```python
from build123d import *

# Parameters (mm, degrees)
BOSS_EXTRUDE1_DEPTH = 36.5
BOSS_EXTRUDE2_DEPTH = 40.35
SKETCH1_4_W         = 22.175
SKETCH1_4_H         = 49.125448028
SKETCH1_4_W_2       = 8.7
SKETCH1_4_H_2       = 18.8
BOSS_EXTRUDE3_DEPTH = 25.8
SKETCH1_5_W         = 8.7
SKETCH1_5_H         = 18.8
BOSS_EXTRUDE4_DEPTH = 20.8
SKETCH1_6_W         = 26.5
SKETCH1_6_H         = 17
BOSS_EXTRUDE5_DEPTH = 7.2
SKETCH1_7_W         = 26.5
SKETCH1_7_H         = 16.1
BOSS_EXTRUDE6_DEPTH = 10
SKETCH1_8_W         = 26.5
SKETCH1_8_H         = 16.1
SKETCH1_8_H_2       = 17
SKETCH1_8_W_2       = 18
SKETCH1_8_H_3       = 43.5
SKETCH1_8_W_3       = 79.7
SKETCH1_8_H_4       = 2.437275986
BOSS_EXTRUDE7_DEPTH = 18.5
SKETCH1_9_W         = 79.7
SKETCH1_9_H         = 2.437275986
SKETCH1_9_W_2       = 26.5
SKETCH1_9_H_2       = 16.1
SKETCH1_9_H_3       = 17
SKETCH1_9_W_3       = 18
SKETCH1_9_H_4       = 43.5
SKETCH1_9_W_4       = 22.175
SKETCH1_9_H_5       = 49.125448028
SKETCH1_9_W_5       = 8.7
SKETCH1_9_H_6       = 18.8
BOSS_EXTRUDE8_DEPTH = 2
BOSS_EXTRUDE9_DEPTH = 2


with BuildPart() as part:
    # Sketch1 → Boss-Extrude1 (new body)
    with BuildSketch(Plane(origin=(0, 0, 0), x_dir=(1, 0, 0), z_dir=(0, 1, 0))):
        Polygon((-41.85, -51), (-39.85, -51), (-39.85, -48.562724014), (-39.85, -28.312724014), (-39.85, 48.562724014), (17.675, 48.562724014), (39.85, 48.562724014), (39.85, -0.562724014), (39.85, -48.562724014), (39.85, -51), (41.85, -51), (41.85, 51), (-41.85, 51), align=None)
    extrude(amount=BOSS_EXTRUDE1_DEPTH)

    # Sketch1_3 → Boss-Extrude2 (add)
    with BuildSketch(Plane(origin=(0, 0, 0), x_dir=(1, 0, 0), z_dir=(0, 1, 0))):
        Polygon((43.85, -51), (41.85, -51), (41.85, 51), (-41.85, 51), (-41.85, -51), (-43.85, -51), (-43.85, 53), (43.85, 53), align=None)
    extrude(amount=BOSS_EXTRUDE2_DEPTH)

    # Sketch1_4 → Boss-Extrude3 (add)
    with BuildSketch(Plane(origin=(0, 0, 0), x_dir=(1, 0, 0), z_dir=(0, 1, 0))):
        with Locations((28.7625, 24)):
            Rectangle(SKETCH1_4_W, SKETCH1_4_H)
        with Locations((28.7625, 24)):
            Rectangle(SKETCH1_4_W_2, SKETCH1_4_H_2, mode=Mode.SUBTRACT)
    extrude(amount=BOSS_EXTRUDE3_DEPTH)

    # Sketch1_5 → Boss-Extrude4 (add)
    with BuildSketch(Plane(origin=(0, 0, 0), x_dir=(1, 0, 0), z_dir=(0, 1, 0))):
        with Locations((28.7625, 24)):
            Rectangle(SKETCH1_5_W, SKETCH1_5_H)
    extrude(amount=BOSS_EXTRUDE4_DEPTH)



with BuildPart() as body_2:
    # Sketch1_6 → Boss-Extrude5 (new body)
    with BuildSketch(Plane(origin=(0, 0, 0), x_dir=(1, 0, 0), z_dir=(0, 1, 0))):
        with Locations((4.25, -38.812724014)):
            Rectangle(SKETCH1_6_W, SKETCH1_6_H)
    extrude(amount=BOSS_EXTRUDE5_DEPTH)


with BuildPart() as body_3:
    # Sketch1_7 → Boss-Extrude6 (new body)
    with BuildSketch(Plane(origin=(0, 0, 0), x_dir=(1, 0, 0), z_dir=(0, 1, 0))):
        with Locations((-24.425, -38.812724014)):
            Rectangle(SKETCH1_7_W, SKETCH1_7_H)
    extrude(amount=BOSS_EXTRUDE6_DEPTH)


with BuildPart() as part_1:
    add(part.part)

    add(body_2.part)  # Boss-Extrude7 merges body 2

    add(body_3.part)  # Boss-Extrude7 merges body 3
    # Sketch1_8 → Boss-Extrude7 (add)
    # profile 1 of 2: a face of its own
    with BuildSketch(Plane(origin=(0, 0, 0), x_dir=(1, 0, 0), z_dir=(0, 1, 0))):
        Polygon((-39.85, -28.312724014), (-39.85, -48.562724014), (39.85, -48.562724014), (39.85, -0.562724014), (17.675, -0.562724014), (17.675, -28.312724014), align=None)
        with Locations((-24.425, -38.812724014)):
            Rectangle(SKETCH1_8_W, SKETCH1_8_H, mode=Mode.SUBTRACT)
        with Locations((4.25, -38.812724014)):
            Rectangle(SKETCH1_8_W, SKETCH1_8_H_2, mode=Mode.SUBTRACT)
        with Locations((28.675, -25.562724014)):
            Rectangle(SKETCH1_8_W_2, SKETCH1_8_H_3, mode=Mode.SUBTRACT)
    # profile 2 of 2: a face of its own
    with BuildSketch(Plane(origin=(0, 0, 0), x_dir=(1, 0, 0), z_dir=(0, 1, 0))):
        with Locations((0, -49.781362007)):
            Rectangle(SKETCH1_8_W_3, SKETCH1_8_H_4)
    extrude(amount=BOSS_EXTRUDE7_DEPTH)

    # Sketch1_9 → Boss-Extrude8 (add)
    # profile 1 of 10: a face of its own
    with BuildSketch(Plane(origin=(0, 0, 0), x_dir=(1, 0, 0), z_dir=(0, 1, 0))):
        with Locations((0, -49.781362007)):
            Rectangle(SKETCH1_9_W, SKETCH1_9_H)
    # profile 2 of 10: a face of its own
    with BuildSketch(Plane(origin=(0, 0, 0), x_dir=(1, 0, 0), z_dir=(0, 1, 0))):
        Polygon((43.85, -51), (41.85, -51), (41.85, 51), (-41.85, 51), (-41.85, -51), (-43.85, -51), (-43.85, 53), (43.85, 53), align=None)
    # profile 3 of 10: a face of its own
    with BuildSketch(Plane(origin=(0, 0, 0), x_dir=(1, 0, 0), z_dir=(0, 1, 0))):
        Polygon((-41.85, -51), (-39.85, -51), (-39.85, -48.562724014), (-39.85, -28.312724014), (-39.85, 48.562724014), (17.675, 48.562724014), (39.85, 48.562724014), (39.85, -0.562724014), (39.85, -48.562724014), (39.85, -51), (41.85, -51), (41.85, 51), (-41.85, 51), align=None)
    # profile 4 of 10: a face of its own
    with BuildSketch(Plane(origin=(0, 0, 0), x_dir=(1, 0, 0), z_dir=(0, 1, 0))):
        Polygon((-39.85, -28.312724014), (-39.85, -48.562724014), (39.85, -48.562724014), (39.85, -0.562724014), (17.675, -0.562724014), (17.675, -28.312724014), align=None)
        with Locations((-24.425, -38.812724014)):
            Rectangle(SKETCH1_9_W_2, SKETCH1_9_H_2, mode=Mode.SUBTRACT)
        with Locations((4.25, -38.812724014)):
            Rectangle(SKETCH1_9_W_2, SKETCH1_9_H_3, mode=Mode.SUBTRACT)
        with Locations((28.675, -25.562724014)):
            Rectangle(SKETCH1_9_W_3, SKETCH1_9_H_4, mode=Mode.SUBTRACT)
    # profile 5 of 10: a face of its own
    with BuildSketch(Plane(origin=(0, 0, 0), x_dir=(1, 0, 0), z_dir=(0, 1, 0))):
        with Locations((-24.425, -38.812724014)):
            Rectangle(SKETCH1_9_W_2, SKETCH1_9_H_2)
    # profile 6 of 10: a face of its own
    with BuildSketch(Plane(origin=(0, 0, 0), x_dir=(1, 0, 0), z_dir=(0, 1, 0))):
        with Locations((4.25, -38.812724014)):
            Rectangle(SKETCH1_9_W_2, SKETCH1_9_H_3)
    # profile 7 of 10: a face of its own
    with BuildSketch(Plane(origin=(0, 0, 0), x_dir=(1, 0, 0), z_dir=(0, 1, 0))):
        with Locations((28.7625, 24)):
            Rectangle(SKETCH1_9_W_4, SKETCH1_9_H_5)
        with Locations((28.7625, 24)):
            Rectangle(SKETCH1_9_W_5, SKETCH1_9_H_6, mode=Mode.SUBTRACT)
    # profile 8 of 10: a face of its own
    with BuildSketch(Plane(origin=(0, 0, 0), x_dir=(1, 0, 0), z_dir=(0, 1, 0))):
        with Locations((28.7625, 24)):
            Rectangle(SKETCH1_9_W_5, SKETCH1_9_H_6)
    # profile 9 of 10: a face of its own
    with BuildSketch(Plane(origin=(0, 0, 0), x_dir=(1, 0, 0), z_dir=(0, 1, 0))):
        Polygon((-39.85, 48.562724014), (-39.85, -28.312724014), (17.675, -28.312724014), (17.675, -0.562724014), (17.675, 48.562724014), align=None)
    # profile 10 of 10: a face of its own
    with BuildSketch(Plane(origin=(0, 0, 0), x_dir=(1, 0, 0), z_dir=(0, 1, 0))):
        with Locations((28.675, -25.562724014)):
            Rectangle(SKETCH1_9_W_3, SKETCH1_9_H_4)
    extrude(amount=-BOSS_EXTRUDE8_DEPTH)

    # Sketch2 → Boss-Extrude9 (add)
    with BuildSketch(Plane(origin=(0, 40.35, 0), x_dir=(1, 0, 0), z_dir=(0, 1, 0))):
        Polygon((-41.85, -51), (-41.85, 51), (41.85, 51), (41.85, -51), (39.85, -51), (39.85, 49), (-39.85, 49), (-39.85, -51), align=None)
    extrude(amount=-BOSS_EXTRUDE9_DEPTH)


solid = part_1.part
```
Geometry: final body of the model. Coordinates: model frame, mm. A direction names the side the tool comes from. Round coordinates to 2 decimals unless told otherwise and drop trailing zeros. Order: outer loops, then holes, each group sorted by start corner. A loop starts at its lowest first (then second) coordinate and runs counter-clockwise, first axis right, second up. Notation, with made-up numbers: M 4.5,70.25 L 21.5,70.25 A6 cw 21.5,80.25 Z; hole C -25,-15.75 d4. An arc over 180 degrees is marked long. One line per item, written item: value.
(1) Cut plane D-D (y = 15.5). Return the cut outline in (x, z) (3 decimals).
Result sheet:
outline: M -43.85,-53 L 43.85,-53 L 43.85,51 L -43.85,51 Z; hole M -39.85,-48.563 L 17.675,-48.563 L 17.675,28.313 L -39.85,28.313 Z; hole M -37.675,30.763 L -11.175,30.763 L -11.175,46.863 L -37.675,46.863 Z; hole M -9,30.313 L 17.5,30.313 L 17.5,47.313 L -9,47.313 Z; hole M 19.675,3.813 L 37.675,3.813 L 37.675,47.313 L 19.675,47.313 Z
(2) Pull-direction query (Y, two-part tool) for faces 3 (the flat face through (-3, 18.5, 29)), 4 (the flat face through (29, 9, 47.313)), 5 (the flat face through (-1, -2, -2)), 6 (the flat face through (0, 36.5, -49)); classes: pulls with the +Y half, pulls with the -Y half, needs draft (parallel to the pull), parting line crosses it, or undercut.
Result sheet:
face 3: pulls with the +Y half
face 4: needs draft
face 5: pulls with the -Y half
face 6: undercut
(3) Pin query (flat end, axial travel): P1, Ø3, axis at x = 30.5, y = 31, coming from the +Z side; P2, Ø2, axis at x = -3.5, y = 38, coming from the +Z side; P3, Ø2, axis at x = 6, z = -40, coming from the +Y side. Return the tip coordinate at first contact, or that it passes through.
Result sheet:
P1: z = -48.56
P2: z = -49
P3: y = 0
(4) Reachability of faces 1 (the flat face through (-43.85, 19, 0)), 2 (the flat face through (29, 20.8, -24)) from +Z, -Z, +X, -X, +Y, -Y: full face, straight path, thin tool, end or side. Return the list, or none.
Result sheet:
face 1: +Z, -Z, -X, +Y, -Y
face 2: +Y
(5) Cut plane C-C (x = -34.5). Return the cut outline in (y, z).
Result sheet:
outline: M -2,-53 L 40.35,-53 L 40.35,-49 L 38.35,-49 L 38.35,-51 L 36.5,-51 L 36.5,-48.56 L 0,-48.56 L 0,28.31 L 18.5,28.31 L 18.5,30.76 L 10,30.76 L 10,46.86 L 18.5,46.86 L 18.5,51 L -2,51 Z
(6) Cut plane A-A (y = 34.5). Return the cut outline in (x, z).
Result sheet:
outline: M -43.85,-53 L 43.85,-53 L 43.85,51 L 39.85,51 L 39.85,-48.56 L -39.85,-48.56 L -39.85,51 L -43.85,51 Z
(7) Line query: probe 1 along X at (y, z) = (15.5, 4) (3 decimals); probe 2 along Z at (x, y) = (-3.5, 8.5); probe 3 along X at (y, z) = (33.5, 34). Output: solid intervals per line, ascending. Write a range as [from, to].
Result sheet:
probe 1: [-43.85, -39.85], [17.675, 19.675], [37.675, 43.85]
probe 2: [-53, -48.56], [28.31, 30.31], [47.31, 51]
probe 3: [-43.85, -39.85], [39.85, 43.85]
